Job drawing, mm, ordinate dimensions from the low corner. One solid piece. Coordinates: 2 decimals unless noted, no trailing zeros. Write each loop counter-clockwise with the first axis right and the second up, starting at its lowest first coordinate (ties: lowest second). Pieces come first, ordered by that corner, then holes. Notation, with made-up numbers: (23, 37) -> (74, 37) arc R5 cw to (74, 41) -> close; hole circle Ø3 at (-37, 55). An arc over 180 degrees is marked (long way). Answer as a JSON object with one key per item and string values. Group by question number.
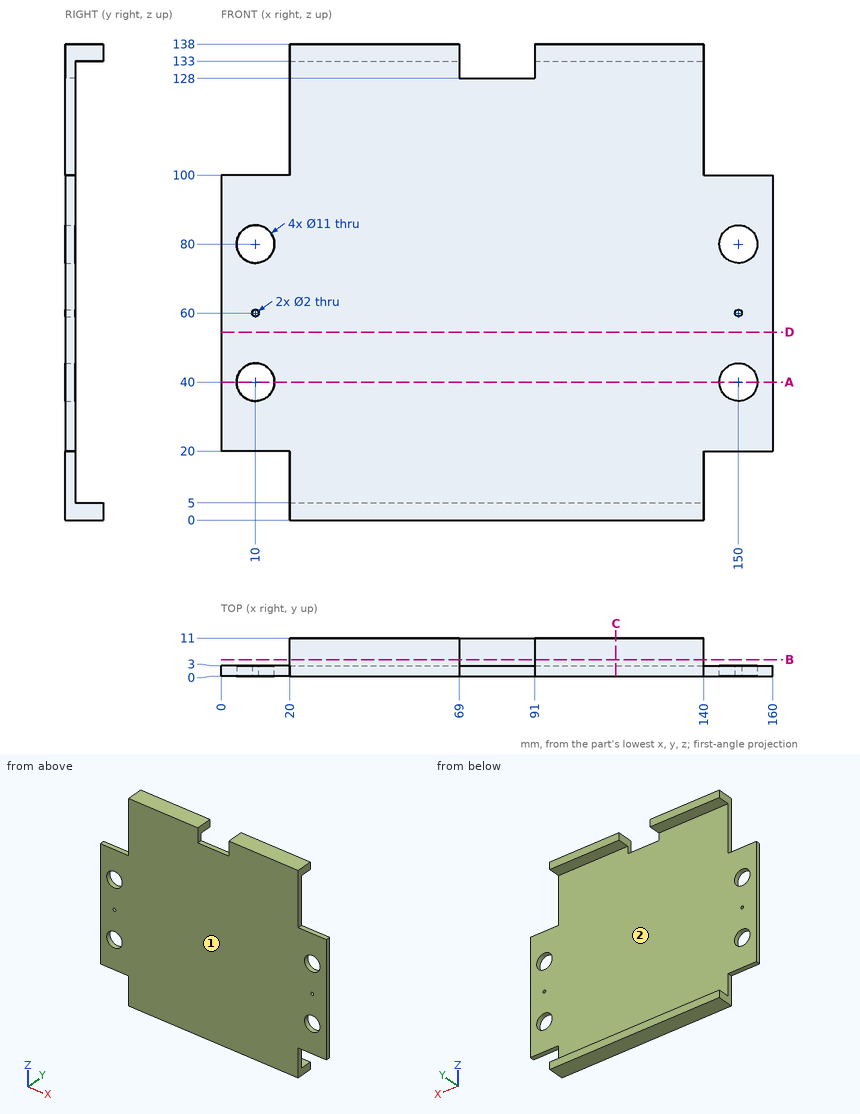
(1) Cut at A-A on z = 40. List the corners of the cut face in (x, y).
(2) Cut at C-C on x = 114.5. List the corners of the cut face in (y, z).
(3) Pin check, flat tips, straight feed: pin 1 (0.9 mm diameter, centred on x = 81, y = 1, fed in from +Z); pin 2 (14.5 mm diameter, centred on x = 10, z = 40, fed in from +Y); pin 3 (3.5 mm diameter, centred on x = 5.5, y = 1.5, fed in from -Z); pin 4 (1.8 mm diameter, centred on x = 10, z = 60, fed in from +Y). Stop position of each tip, or through.
(4) Pull direction Z, two halves, no side cores. Call the marked faces 1 and 2: released by +Z, released by -Z, zero draft, split by the parting line, or undercut.
(5) Wall check: probe 1 along X at (y, z) = (0.9, 60); probe 2 along X at (y, z) = (0.6, 80); probe 3 along Z at (x, y) = (150, 0.75). Give the ranges that are in metal, low to high.
(6) Cut at B-B on y = 4.75. List the corners of the cut face in (x, z), plus the area to 3 significant figures.
(7) Cut at D-D on z = 54.5. List the corners of the cut face in (x, y), plus the area to 3 significant figures.
Results found:
{
 "1": {"outline": "(0, 0) -> (4.5, 0) -> (4.5, 3) -> (0, 3) -> close; (15.5, 0) -> (144.5, 0) -> (144.5, 3) -> (15.5, 3) -> close; (155.5, 0) -> (160, 0) -> (160, 3) -> (155.5, 3) -> close"},
 "2": {"outline": "(0, 0) -> (11, 0) -> (11, 5) -> (3, 5) -> (3, 133) -> (11, 133) -> (11, 138) -> (0, 138) -> close"},
 "3": {"pin 1": "stops at z = 128", "pin 2": "stops at y = 3", "pin 3": "stops at z = 20", "pin 4": "passes through"},
 "4": {"face 1": "zero draft", "face 2": "undercut"},
 "5": {"probe 1": "x = 0 to 9, 11 to 149, 151 to 160", "probe 2": "x = 0 to 4.5, 15.5 to 144.5, 155.5 to 160", "probe 3": "z = 20 to 34.5, 45.5 to 59, 61 to 74.5, 85.5 to 100"},
 "6": {"outline": "(20, 0) -> (140, 0) -> (140, 5) -> (20, 5) -> close; (20, 133) -> (69, 133) -> (69, 138) -> (20, 138) -> close; (91, 133) -> (140, 133) -> (140, 138) -> (91, 138) -> close", "area": "1,090 mm²"},
 "7": {"outline": "(0, 0) -> (160, 0) -> (160, 3) -> (0, 3) -> close", "area": "480 mm²"}
}
